The figure shows three views and two pictorial views of one solid part (mm, origin at its lowest corner). Answer the questions. A direction names the side the tool comes from. Round coordinates to 2 decimals unless told otherwise and drop trailing zeros. Write each loop counter-clockwise with the first axis right and the second up, starting at its lowest first coordinate (ties: lowest second). Pieces come first, ordered by that corner, then holes. Notation, with made-up numbers: M 5,35.25 L 25,35.25 A13 cw 25,51.25 Z; hole C 33.25,-27.5 d8. An arc over 180 degrees is marked long. Answer in a Markdown table with one row per item.
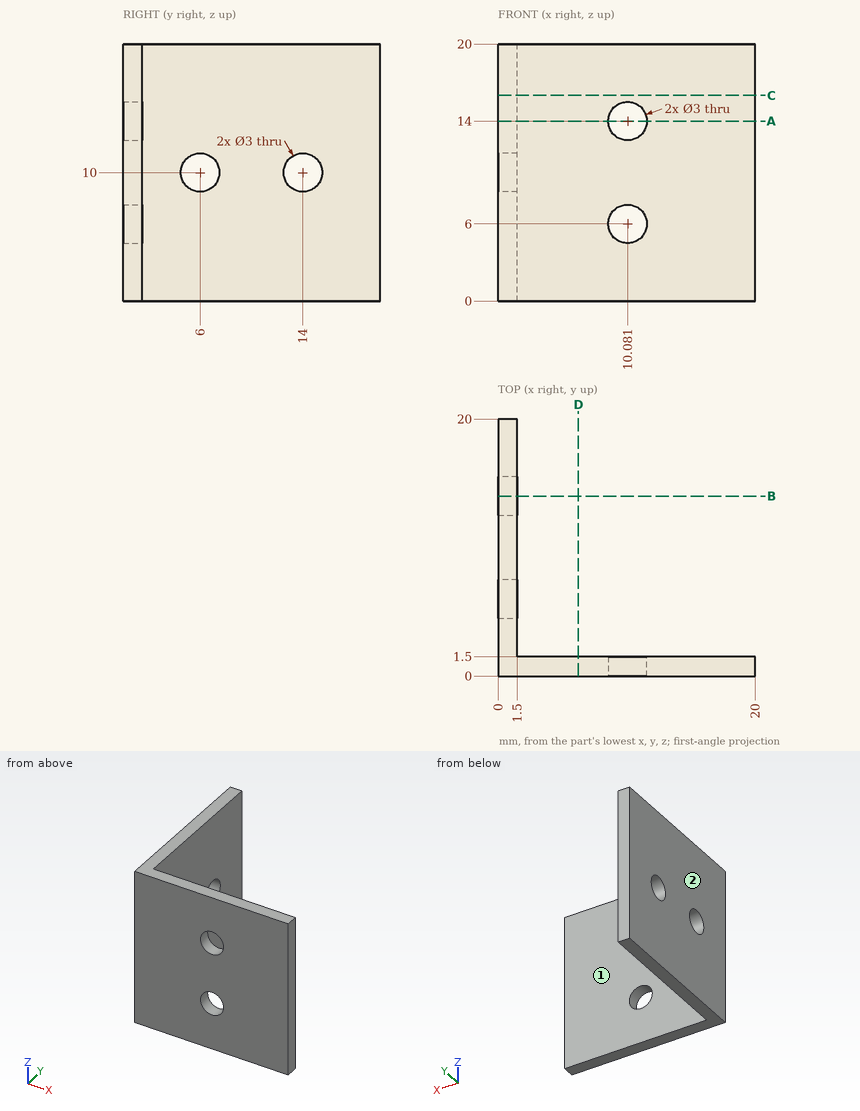
1. Given pin 1 (1.8 mm diameter, centred on x = 10.08, z = 6, fed in from -Y); pin 2 (9 mm diameter, centred on y = 14.5, z = 15, fed in from +X); pin 3 (9 mm diameter, centred on x = 12, z = 10, fed in from +Y), each flat-ended and moving along its own axis, determine where each tip first touches the part or whether it passes through.
Calculated:
| item | result |
|---|---|
| pin 1 | passes through |
| pin 2 | stops at x = 1.5 |
| pin 3 | stops at y = 1.5 |
2. The part is cut by section A-A (z = 14). Determine the outline of the cut face in (x, y).
Calculated:
| item | result |
|---|---|
| outline | M 0,0 L 8.58,0 L 8.58,1.5 L 1.5,1.5 L 1.5,20 L 0,20 Z; M 11.58,0 L 20,0 L 20,1.5 L 11.58,1.5 Z |
3. A tool of negligible diameter and unlimited length cuts with its end or side. For the marked faces 1 and 2, from which of +Z, -Z, +X, -X, +Y, -Y can it reach the whole face along a straight path? Write none if from no direction.
Calculated:
| item | result |
|---|---|
| face 1 | +Z, -Z, +X, +Y |
| face 2 | +Z, -Z, -X, +Y, -Y |
4. The part is cut by section B-B (y = 14). Determine the outline of the cut face in (x, z).
Calculated:
| item | result |
|---|---|
| outline | M 0,0 L 1.5,0 L 1.5,8.5 L 0,8.5 Z; M 0,11.5 L 1.5,11.5 L 1.5,20 L 0,20 Z |
5. Consider line 1 along Z through (x, y) = (0.5, 6); line 2 along Y through (x, z) = (9.75, 12). Determine where each line is inside the solid, lowest interval first. Write a range as from..to.
Calculated:
| item | result |
|---|---|
| line 1 | z = 0..8.5, 11.5..20 |
| line 2 | y = 0..1.5 |
6. The part is cut by section C-C (z = 16). Determine the outline of the cut face in (x, y).
Calculated:
| item | result |
|---|---|
| outline | M 0,0 L 20,0 L 20,1.5 L 1.5,1.5 L 1.5,20 L 0,20 Z |
7. The part is cut by section D-D (x = 6.25). Determine the outline of the cut face in (y, z).
Calculated:
| item | result |
|---|---|
| outline | M 0,0 L 1.5,0 L 1.5,20 L 0,20 Z |
